```python
from build123d import *

# Parameters (mm, degrees)
F0_W      = 54
F0_H      = 36
F1_DEPTH  = 44
F2_W      = 40
F2_H      = 29
F3_DEPTH  = 36
F4_W      = 11
F4_H      = 36
F5_DEPTH  = 7
F6_W      = 7
F6_H      = 18
F7_DEPTH  = 7
F8_W      = 11
F8_H      = 36
F9_DEPTH  = 7
F10_W     = 7
F10_H     = 18
F11_DEPTH = 7
F12_R     = 15
F13_DEPTH = 22
F14_R     = 10
F15_DEPTH = 40
F17_DEPTH = 7


with BuildPart() as f1:
    # F0 (on Top) → F1 (new body)
    with BuildSketch(Plane.XY):
        with Locations((12.5230278373, -18.4144742489)):
            Rectangle(F0_W, F0_H)
    extrude(amount=F1_DEPTH)

    # F2 (on face) → F3 (cut)
    with BuildSketch(Plane.XZ.offset(36.4144742489)):
        with Locations((12.1546047553, 29.5)):
            Rectangle(F2_W, F2_H)
    extrude(amount=-F3_DEPTH, mode=Mode.SUBTRACT)

    # F4 (on face) → F5 (join)
    with BuildSketch(Plane.XY.offset(44)):
        with Locations((45.0230278373, -18.4144742489)):
            Rectangle(F4_W, F4_H)
    extrude(amount=-F5_DEPTH)

    # F6 (on face) → F7 (cut)
    with BuildSketch(Plane.XY.offset(44)):
        with Locations((47.0230278373, -18.8289485723)):
            Rectangle(F6_W, F6_H)
    extrude(amount=-F7_DEPTH, mode=Mode.SUBTRACT)

    # F8 (on face) → F9 (join)
    with BuildSketch(Plane.XY.offset(44)):
        with Locations((-19.9769721627, -18.4144742489)):
            Rectangle(F8_W, F8_H)
    extrude(amount=-F9_DEPTH)

    # F10 (on face) → F11 (cut)
    with BuildSketch(Plane.XY.offset(44)):
        with Locations((-21.9769721627, -18.8289485723)):
            Rectangle(F10_W, F10_H)
    extrude(amount=-F11_DEPTH, mode=Mode.SUBTRACT)

    # F12 (on face) → F13 (join)
    with BuildSketch(Plane.XY.offset(15)):
        with Locations((11.9901327416, -18.3494538069)):
            Circle(F12_R)
    extrude(amount=F13_DEPTH)

    # F14 (on face) → F15 (cut)
    with BuildSketch(Plane.XY.offset(37)):
        with Locations((11.9901327416, -18.3494538069)):
            Circle(F14_R)
    extrude(amount=-F15_DEPTH, mode=Mode.SUBTRACT)

    # F16 (on face) → F17 (cut)
    with BuildSketch(Plane.XY.offset(37)):
        with BuildLine():
            ThreePointArc((17.0230269432, -4.2189911126), (12.0250223229, -3.349494383), (7.0230269432, -4.1957313288))
            Line((7.0230269432, -4.1957313288), (7.0230269432, -9.6702914056))
            ThreePointArc((7.0230269432, -9.6702914056), (12.0281157852, -8.3495259427), (17.0230269432, -9.7082747232))
            Line((17.0230269432, -9.7082747232), (17.0230269432, -4.2189911126))
        make_face()
        with BuildLine():
            Line((7.0230269432, -27.0286162081), (7.0230269432, -32.503176285))
            ThreePointArc((7.0230269432, -32.503176285), (12.0250223229, -33.3494132307), (17.0230269432, -32.4799165012))
            Line((17.0230269432, -32.4799165012), (17.0230269432, -26.9906328905))
            ThreePointArc((17.0230269432, -26.9906328905), (12.0281157852, -28.349381671), (7.0230269432, -27.0286162081))
        make_face()
    extrude(amount=-F17_DEPTH, mode=Mode.SUBTRACT)


solid = f1.part
```
Geometry: final body of the model. Coordinates: model frame, mm. A direction names the side the tool comes from. Coordinates: 2 decimals unless noted, no trailing zeros. Write each loop counter-clockwise with the first axis right and the second up, starting at its lowest first coordinate (ties: lowest second). Pieces come first, ordered by that corner, then holes. Notation, with made-up numbers: M -8.5,-34.5 L 20.5,-34.5 A22 ccw 20.5,-19.5 Z; hole C -32.75,2.25 d8. An arc over 180 degrees is marked long. Use CSV: the item, a comma, the result in double quotes. Start each with the question number.
1. First-contact query: P1, Ø8, axis at y = -16, z = 32, coming from the +X side; P2, Ø5, axis at x = 10.5, y = -6.5, coming from the +Z side; P3, Ø11, axis at x = 23.5, y = -13.5, coming from the +Z side. Flat tips, straight axial feed; report the tip coordinate or a pass-through.
2. Reachability of faces 5 (the face through (25.85, -24.09, 25.85)), 6 (the face through (-22, -9.829, 41)), 7 (the face through (12, -6, 30)) from +Z, -Z, +X, -X, +Y, -Y: full face, straight path, thin tool, end or side. Return the list, or none.
3. Cut plane B-B on z = 33.5. Return the cut outline in (x, y), plus the area to 3 significant figures.
4. Cut plane A-A on x = 44.5. Return the cut outline in (y, z), plus the area to 3 significant figures.
5. Cut plane D-D on z = 40. Return the cut outline in (x, y).
6. Ray query, probe 1 along X at (y, z) = (-2.5, 20.5); probe 2 along X at (y, z) = (-29.5, 15.5); probe 3 along X at (y, z) = (-15.5, 16). Return the intervals inside material, ascending.
7. Mould query, pull axis Y, two halves, no side actions, for faces 1 (the face through (47, -9.829, 41)), 2 (the face through (12, -36.414, 13)), 3 (the face through (-18.477, -19, 41)), 4 (the face through (1, -18, 37)). Classes: pulls with the +Y half, pulls with the -Y half, needs draft (parallel to the pull), parting line crosses it, or undercut.
8. Cut plane C-C on y = -2.5. Return the cut outline in (x, z).
Entries:
1,P1,"x = 39.52"
1,P2,"z = 30"
1,P3,"z = 37"
2,face 5,"+Z"
2,face 6,"+Z, -Z, -X"
2,face 7,"+Z, +Y, -Y"
3,outline,"M -14.48,-36.41 L -7.85,-36.41 L -7.85,-0.41 L -14.48,-0.41 Z; M 7.02,-32.5 L 7.02,-27.03 A10 cw 7.02,-9.67 L 7.02,-4.2 A15 ccw Z; M 17.02,-32.48 A15 ccw 17.02,-4.22 L 17.02,-9.71 A10 cw 17.02,-26.99 Z; M 32.15,-36.41 L 39.52,-36.41 L 39.52,-0.41 L 32.15,-0.41 Z"
3,area,"794 mm²"
4,outline,"M -36.41,37 L -27.83,37 L -27.83,44 L -36.41,44 Z; M -9.83,37 L -0.41,37 L -0.41,44 L -9.83,44 Z"
4,area,"126 mm²"
5,outline,"M -25.48,-36.41 L -7.85,-36.41 L -7.85,-0.41 L -25.48,-0.41 L -25.48,-9.83 L -18.48,-9.83 L -18.48,-27.83 L -25.48,-27.83 Z; M 32.15,-36.41 L 50.52,-36.41 L 50.52,-27.83 L 43.52,-27.83 L 43.52,-9.83 L 50.52,-9.83 L 50.52,-0.41 L 32.15,-0.41 Z"
6,probe 1,"-14.48 to -7.85, 32.15 to 39.52"
6,probe 2,"-14.48 to -7.85, 1.96 to 22.02, 32.15 to 39.52"
6,probe 3,"-14.48 to -7.85, -2.74 to 2.4, 21.58 to 26.72, 32.15 to 39.52"
7,face 1,"undercut"
7,face 2,"pulls with the -Y half"
7,face 3,"undercut"
7,face 4,"needs draft"
8,outline,"M -25.48,37 L -14.48,37 L -14.48,0 L 39.52,0 L 39.52,37 L 50.52,37 L 50.52,44 L 32.15,44 L 32.15,15 L -7.85,15 L -7.85,44 L -25.48,44 Z"
